Input: part model. Units: mm. Frame: model coordinates. Face numbers are marked on the shaded views. Coordinates: 2 decimals unless noted, no trailing zeros. Order: outer loops, then holes, each group sorted by start corner. A loop starts at its lowest first (then second) coordinate and runs counter-clockwise, first axis right, second up.
from build123d import *

# Parameters (mm, degrees)
BOX001_W     = 20
BOX001_H     = 200
BOX001_DEPTH = 30
BOX002_W     = 200
BOX002_H     = 10
BOX002_DEPTH = 20
BOX003_W     = 200
BOX003_H     = 10
BOX003_DEPTH = 20
BOX004_W     = 300
BOX004_H     = 200
BOX004_DEPTH = 5
BOX_W        = 200
BOX_H        = 200
BOX_DEPTH    = 5


with BuildPart() as cube001:
    # Box001 → Box001 (new body)
    with BuildSketch(Plane.XY):
        with Locations((10, 100)):
            Rectangle(BOX001_W, BOX001_H)
    extrude(amount=BOX001_DEPTH)


with BuildPart() as cube002:
    # Box002 → Box002 (new body)
    with BuildSketch(Plane(origin=(100, 190, -20), x_dir=(1, 0, 0), z_dir=(0, 0, 1))):
        with Locations((100, 5)):
            Rectangle(BOX002_W, BOX002_H)
    extrude(amount=BOX002_DEPTH)


with BuildPart() as cube003:
    # Box003 → Box003 (new body)
    with BuildSketch(Plane(origin=(100, 0, -20), x_dir=(1, 0, 0), z_dir=(0, 0, 1))):
        with Locations((100, 5)):
            Rectangle(BOX003_W, BOX003_H)
    extrude(amount=BOX003_DEPTH)


with BuildPart() as cube004:
    # Box004 → Box004 (new body)
    with BuildSketch(Plane.XY):
        with Locations((150, 100)):
            Rectangle(BOX004_W, BOX004_H)
    extrude(amount=BOX004_DEPTH)


with BuildPart() as fusion:
    # Box → Box (new body)
    with BuildSketch(Plane(origin=(100, 0, -20), x_dir=(1, 0, 0), z_dir=(0, 0, 1))):
        with Locations((100, 100)):
            Rectangle(BOX_W, BOX_H)
    extrude(amount=BOX_DEPTH)

    # Fusion: union Cube001, Cube002, Cube003, Cube004
    add(cube001.part)
    add(cube002.part)
    add(cube003.part)
    add(cube004.part)


solid = fusion.part
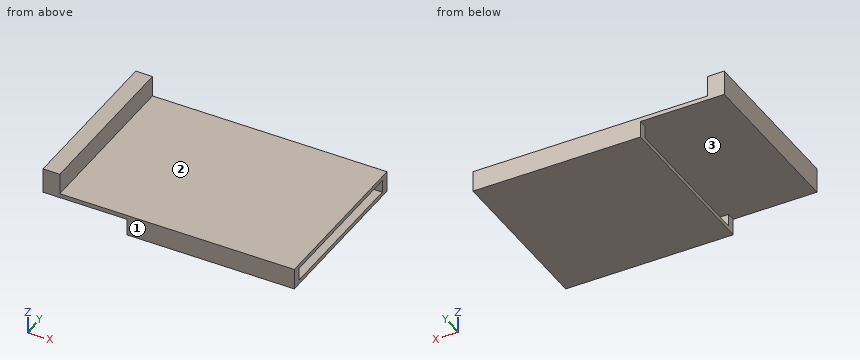
Item 1: Draft query along Y for the marked faces 1, 2 and 3. Return one class per face: pulls with the +Y half, pulls with the -Y half, needs draft (parallel to the pull), parting line crosses it, or undercut.
Response values:
face 1: pulls with the -Y half
face 2: needs draft
face 3: undercut
Item 2: Pin query (flat end, axial travel): pin 1 Ø6 at (x, y) = (76, 133) entering from -Z; pin 2 Ø5 at (x, y) = (218, 28) entering from +Z; pin 3 Ø10 at (y, z) = (165, -5.5) entering from +X; pin 4 Ø1 at (y, z) = (148, 8) entering from +X. Return the tip coordinate at first contact, or that it passes through.
Response values:
pin 1: stops at z = 0
pin 2: stops at z = 5
pin 3: passes through
pin 4: stops at x = 20
Item 3: Ray query, probe 1 along Z at (x, y) = (142.5, 21.5); probe 2 along Y at (x, z) = (107.5, -4); probe 3 along X at (y, z) = (112, 9). Return the intervals inside material, ascending.
Response values:
probe 1: z = -20 to -15, 0 to 5
probe 2: y = 0 to 10, 190 to 200
probe 3: x = 0 to 20
Item 4: Cut plane C-C on y = 131. Return loops of the section in (x, z), then the cut area to 3 significant figures.
Response values:
outline: (0, 0) - (300, 0) - (300, 5) - (20, 5) - (20, 30) - (0, 30) - close; (100, -20) - (300, -20) - (300, -15) - (100, -15) - close
area: 3,000 mm2
Item 5: Cut plane A-A on z = -11.5. Return loops of the section in (x, y).
Response values:
outline: (100, 0) - (300, 0) - (300, 10) - (100, 10) - close; (100, 190) - (300, 190) - (300, 200) - (100, 200) - close
Item 6: Cut plane D-D on z = 13.5. Return loops of the section in (x, y), then the cut area to 3 significant figures.
Response values:
outline: (0, 0) - (20, 0) - (20, 200) - (0, 200) - close
area: 4,000 mm2
Item 7: Cut plane B-B on x = 279.5. Return loops of the section in (y, z), then the cut area to 3 significant figures.
Response values:
outline: (0, -20) - (200, -20) - (200, 5) - (0, 5) - close; hole (10, -15) - (190, -15) - (190, 0) - (10, 0) - close
area: 2,300 mm2
